from build123d import *

# Parameters (mm, degrees)
SKETCH1_W                 = 47
SKETCH1_H                 = 65
BOSS_EXTRUDE1_DEPTH       = 3
F_3_0MM_DOWEL_HOLE1_D     = 3
F_3_0MM_DOWEL_HOLE1_DEPTH = 4
F_3_0MM_DOWEL_HOLE1_TIP   = 0.901290929


with BuildPart() as part:
    # Sketch1 → Boss-Extrude1 (new body)
    with BuildSketch(Plane.XY):
        Rectangle(SKETCH1_W, SKETCH1_H)
    extrude(amount=BOSS_EXTRUDE1_DEPTH)

    # Ø3.0mm Dowel Hole1
    with Locations(Plane.XY.offset(3)):
        with Locations((-13, -29), (13, -29), (13, 29), (-13, 29)):
            Hole(F_3_0MM_DOWEL_HOLE1_D / 2, depth=F_3_0MM_DOWEL_HOLE1_DEPTH)
            with Locations((0, 0, -(F_3_0MM_DOWEL_HOLE1_DEPTH + F_3_0MM_DOWEL_HOLE1_TIP / 2))):  # 118° drill point
                Cone(0, F_3_0MM_DOWEL_HOLE1_D / 2, F_3_0MM_DOWEL_HOLE1_TIP, mode=Mode.SUBTRACT)


solid = part.part
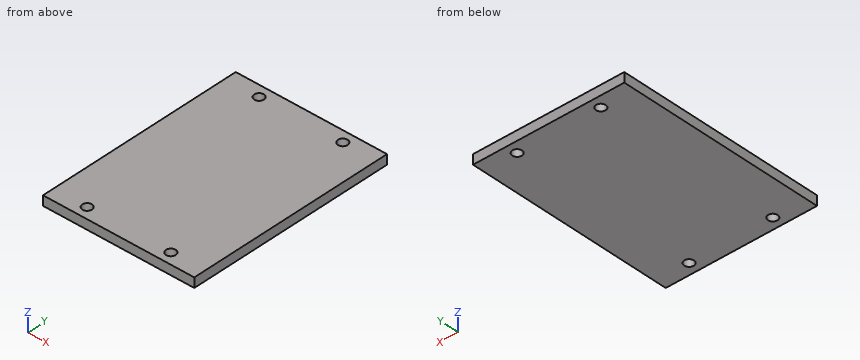
Could you check a few things on this model? Use its own coordinates, in mm. Round coordinates to 2 decimals unless told otherwise and drop trailing zeros. Order: outer loops, then holes, each group sorted by start corner. A loop starts at its lowest first (then second) coordinate and runs counter-clockwise, first axis right, second up.
(1) I'm going to push a flat-ended pin straight in: pin 1 (3 mm diameter, centred on x = 0.5, y = 2, fed in from -Z). Where does the tip first touch, or does it pass through?
Response values:
pin 1: stops at z = 0
(2) Please list where these lines run through material, in increasing order: line 1 along Y through (x, z) = (-13, 1.65); line 2 along Y through (x, z) = (-14, 0.3); line 3 along X through (y, z) = (29.5, 2).
Response values:
line 1: y = -32.5 to -30.5, -27.5 to 27.5, 30.5 to 32.5
line 2: y = -32.5 to -30.12, -27.88 to 27.88, 30.12 to 32.5
line 3: x = -23.5 to -14.41, -11.59 to 11.59, 14.41 to 23.5
(3) Imagine slicing it at A-A (x = 13). Write out the boundary of the cut face in (y, z).
Response values:
outline: (-32.5, 0) - (-30.5, 0) - (-30.5, 3) - (-32.5, 3) - close; (-27.5, 0) - (27.5, 0) - (27.5, 3) - (-27.5, 3) - close; (30.5, 0) - (32.5, 0) - (32.5, 3) - (30.5, 3) - close
(4) Imagine slicing it at B-B (y = -29). Write out the boundary of the cut face in (x, z), plus the area to 3 significant figures.
Response values:
outline: (-23.5, 0) - (-14.5, 0) - (-14.5, 3) - (-23.5, 3) - close; (-11.5, 0) - (11.5, 0) - (11.5, 3) - (-11.5, 3) - close; (14.5, 0) - (23.5, 0) - (23.5, 3) - (14.5, 3) - close
area: 123 mm2
